Verification items for the finished model (mm, model axes). Face numbers are marked on the shaded views. A direction names the side the tool comes from. Give positions to 0.01 mm unless a question says otherwise; leave off trailing zeros. Write each loop counter-clockwise with the first axis right and the second up, starting at its lowest first coordinate (ties: lowest second). Pieces come first, ordered by that corner, then holes. Notation, with made-up numbers: (-35, 41) -> (-13, 41) arc R36 cw to (-13, 77) -> close; hole circle Ø4 at (65.5, -37). An arc over 180 degrees is marked (long way). Use one line per item in the form item = value. Start each with the question number.
(1) Section check D-D, the plane x = -24. Record the cut outline in (y, z), plus the area to 3 significant figures.
(2) Section check C-C, the plane x = 24.5. Record the cut outline in (y, z).
(3) Scan lines: L1, parallel to X at y = -16, z = 45; L2, parallel to Z at x = -26, y = 0; L3, parallel to Z at x = 24, y = 0. Record each from-to range of solid material in increasing order.
(4) Set-up check for the marked faces 1, 2 and 3: record each of +Z, -Z, +X, -X, +Y, -Y from which the full face is reachable in a straight line by a thin tool's end or side.
(5) Release check for a two-part mould opening along Z. For the marked faces 4, 5 and 6 record: pulls with the +Z half, pulls with the -Z half, needs draft (parallel to the pull), parting line crosses it, or undercut.
(6) Section check A-A, the plane x = 0. Record the cut outline in (y, z).
(7) Depth check by flat-ended pin: pin 1 Ø20 at (y, z) = (4, 18) entering from +X; pin 2 Ø10 at (y, z) = (-3.5, 17.5) entering from +X; pin 3 Ø15.5 at (x, z) = (0, 25) entering from -Y; pin 4 Ø20 at (x, y) = (-7.5, -0.5) entering from +Z. Enter the tip coordinate at first touch or a pass-through.
(8) Section check B-B, the plane y = 0. Record the cut outline in (x, z).
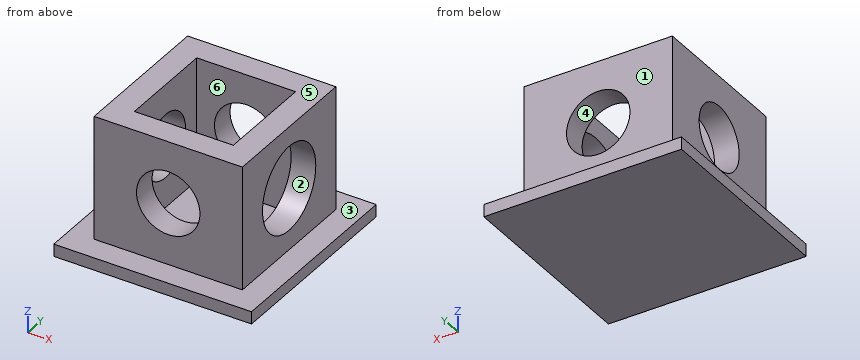
from build123d import *

# Parameters (mm, degrees)
F0_W      = 60
F0_H      = 60
F2_DEPTH  = 50
F1_W      = 40
F1_H      = 40
F3_DEPTH  = 50
F4_R      = 12.84
F5_DEPTH  = 60
F6_R      = 12.84
F7_DEPTH  = 10
F8_R      = 17.1
F9_DEPTH  = 25
F10_W     = 80
F10_H     = 80
F11_DEPTH = 5


with BuildPart() as f2:
    # F0 (on Top) → F2 (new body)
    with BuildSketch(Plane.XY):
        Rectangle(F0_W, F0_H)
    extrude(amount=F2_DEPTH)

    # F1 (on Top) → F3 (cut)
    with BuildSketch(Plane.XY):
        Rectangle(F1_W, F1_H)
    extrude(amount=F3_DEPTH, mode=Mode.SUBTRACT)

    # F4 (on face) → F5 (cut)
    with BuildSketch(Plane.XZ.offset(30)):
        with Locations((0, 25)):
            Circle(F4_R)
    extrude(amount=-F5_DEPTH, mode=Mode.SUBTRACT)

    # F6 (on face) → F7 (cut)
    with BuildSketch(Plane(origin=(-30, 0, 0), x_dir=(0, -1, 0), z_dir=(-1, 0, 0))):
        with Locations((0, 25)):
            Circle(F6_R)
    extrude(amount=-F7_DEPTH, mode=Mode.SUBTRACT)

    # F8 (on face) → F9 (cut)
    with BuildSketch(Plane.YZ.offset(30)):
        with Locations((0, 25)):
            Circle(F8_R)
    extrude(amount=-F9_DEPTH, mode=Mode.SUBTRACT)

    # F10 (on Top) → F11 (join)
    with BuildSketch(Plane.XY):
        Rectangle(F10_W, F10_H)
    extrude(amount=-F11_DEPTH)


solid = f2.part
Completed:
q1.outline = (-40, -5) -> (40, -5) -> (40, 0) -> (30, 0) -> (30, 50) -> (-30, 50) -> (-30, 0) -> (-40, 0) -> close; hole circle Ø25.68 at (0, 25)
q1.area = 2,880 mm²
q2.outline = (-40, -5) -> (40, -5) -> (40, 0) -> (30, 0) -> (30, 50) -> (-30, 50) -> (-30, 0) -> (-40, 0) -> close; hole circle Ø34.2 at (0, 25)
q3.L1 = -30 to -20, 20 to 30
q3.L2 = -5 to 12.16, 37.84 to 50
q3.L3 = -5 to 7.9, 42.1 to 50
q4.face_1 = +Z, +X, -X, +Y
q4.face_2 = +X
q4.face_3 = +Z
q5.face_4 = undercut
q5.face_5 = pulls with the +Z half
q5.face_6 = needs draft
q6.outline = (-40, -5) -> (40, -5) -> (40, 0) -> (30, 0) -> (30, 12.16) -> (20, 12.16) -> (20, 0) -> (-20, 0) -> (-20, 12.16) -> (-30, 12.16) -> (-30, 0) -> (-40, 0) -> close; (-30, 37.84) -> (-20, 37.84) -> (-20, 50) -> (-30, 50) -> close; (20, 37.84) -> (30, 37.84) -> (30, 50) -> (20, 50) -> close
q7.pin_1 = 30
q7.pin_2 = -20
q7.pin_3 = through
q7.pin_4 = 0
q8.outline = (-40, -5) -> (40, -5) -> (40, 0) -> (30, 0) -> (30, 7.9) -> (20, 7.9) -> (20, 0) -> (-20, 0) -> (-20, 12.16) -> (-30, 12.16) -> (-30, 0) -> (-40, 0) -> close; (-30, 37.84) -> (-20, 37.84) -> (-20, 50) -> (-30, 50) -> close; (20, 42.1) -> (30, 42.1) -> (30, 50) -> (20, 50) -> close
